Input: part model. Units: mm. Frame: model coordinates. A direction names the side the tool comes from. Round coordinates to 2 decimals unless told otherwise and drop trailing zeros. Order: outer loops, then holes, each group sorted by start corner. A loop starts at its lowest first (then second) coordinate and runs counter-clockwise, first axis right, second up. Notation, with made-up numbers: M -9,-34 L -3,-34 A19 ccw -3,1 Z; hole C 81.25,-18 d2. An arc over 180 degrees is marked long. One line per question, with ' | ' between items.
```python
from build123d import *

# Parameters (mm, degrees)
BOSS_EXTRUDE1_DEPTH = 2


with BuildPart() as part:
    # Model → Boss-Extrude1 (new body)
    with BuildSketch(Plane.XY):
        with BuildLine():
            Line((11, 2), (11, 5))
            ThreePointArc((11, 5), (10.707106781, 5.707106781), (10, 6))
            Line((10, 6), (8, 6))
            Line((8, 6), (8, 5))
            ThreePointArc((8, 5), (7, 3), (6, 5))
            Line((6, 5), (6, 6))
            Line((6, 6), (3, 6))
            Line((3, 6), (3, 5))
            ThreePointArc((3, 5), (2, 3), (1, 5))
            Line((1, 5), (1, 6))
            Line((1, 6), (-1, 6))
            ThreePointArc((-1, 6), (-1.707106781, 5.707106781), (-2, 5))
            Line((-2, 5), (-2, 2))
            Line((-2, 2), (0, 2))
            Line((0, 2), (0, 0))
            Line((0, 0), (9, 0))
            Line((9, 0), (9, 2))
            Line((9, 2), (11, 2))
        make_face()
    extrude(amount=BOSS_EXTRUDE1_DEPTH)


solid = part.part
```
Item 1: Section query B-B, the plane z = 0.75. Return loops of the section in (x, y), plus the area to 3 significant figures.
Report:
outline: M -2,2 L 0,2 L 0,0 L 9,0 L 9,2 L 11,2 L 11,5 A1 ccw 10,6 L 8,6 L 8,5 A1.25 cw long 6,5 L 6,6 L 3,6 L 3,5 A1.25 cw long 1,5 L 1,6 L -1,6 A1 ccw -2,5 Z | area: 57.2 mm²
Item 2: Section query C-C, the plane x = 7. Return loops of the section in (y, z).
Report:
outline: M 0,0 L 3,0 L 3,2 L 0,2 Z
Item 3: First-contact query: pin 1 (1.5 mm diameter, centred on x = 8, y = 4.5, fed in from -Z); pin 2 (0.8 mm diameter, centred on y = 5.5, z = 0.5, fed in from +X) (3 decimals); pin 3 (0.6 mm diameter, centred on x = 9.5, z = 1, fed in from -Y); pin 4 (0.8 mm diameter, centred on y = 5.5, z = 0.5, fed in from -X) (3 decimals). Flat tips, straight axial feed; report the tip coordinate or a pass-through.
Report:
pin 1: z = 0 | pin 2: x = 10.995 | pin 3: y = 2 | pin 4: x = -1.995
Item 4: Access query for faces 1 (the flat face through (0, 1, 1)), 2 (the flat face through (11, 3, 1)), 3 (the flat face through (10, 2, 1)), 4 (the cylindrical face through (10.715, 5.699, 0.986)), 5 (the flat face through (6, 5.5, 1)). Directions: +Z, -Z, +X, -X, +Y, -Y. A direction counts if a zero-diameter tool reaches every point of the face in a straight line with its end or side. Return the directions, or none.
Report:
face 1: +Z, -Z, -X, -Y | face 2: +Z, -Z, +X, +Y, -Y | face 3: +Z, -Z, +X, -Y | face 4: +Z, -Z, +X, +Y | face 5: +Z, -Z, +Y
Item 5: Section query D-D, the plane y = 0.45. Return loops of the section in (x, z), plus the area to 3 significant figures.
Report:
outline: M 0,0 L 9,0 L 9,2 L 0,2 Z | area: 18.0 mm²
Item 6: Line query: line 1 along X through (y, z) = (4.25, 1.2); line 2 along X through (y, z) = (1.15, 0.3); line 3 along X through (y, z) = (3.65, 0.4). Output: solid intervals per line, ascending. Write a range as from..to.
Report:
line 1: -2..0.75, 3.25..5.75, 8.25..11 | line 2: 0..9 | line 3: -2..0.9, 3.1..5.9, 8.1..11
Item 7: Mould query, pull axis Y, two halves, no side actions, for faces 6 (the flat face through (0, 6, 1)), 7 (the cylindrical face through (7, 3, 1)), 8 (the flat face through (-1, 2, 1)), 9 (the flat face through (9, 1, 1)). Classes: +Y half, -Y half, draft (parallel to the pull), parting line (faces both ways), or undercut.
Report:
face 6: +Y half | face 7: undercut | face 8: -Y half | face 9: draft
Item 8: Section query A-A, the plane y = 4.25. Return loops of the section in (x, z).
Report:
outline: M -2,0 L 0.75,0 L 0.75,2 L -2,2 Z; M 3.25,0 L 5.75,0 L 5.75,2 L 3.25,2 Z; M 8.25,0 L 11,0 L 11,2 L 8.25,2 Z
